from build123d import *

# Parameters (mm, degrees)
BOSS_EXTRUDE1_DEPTH     = 80
CUT_EXTRUDE1_DEPTH      = 206.243757518
CUT_EXTRUDE1_DEPTH_BACK = 206.243757518
SKETCH2_R               = 4
SKETCH5_W               = 15
SKETCH5_H               = 15
BOSS_EXTRUDE2_DEPTH     = 90
CUT_EXTRUDE2_DEPTH      = 230
CUT_EXTRUDE2_DEPTH_BACK = 10
SKETCH6_R               = 4
CUT_EXTRUDE3_DEPTH      = 80
CUT_EXTRUDE3_DEPTH_BACK = 90
SKETCH8_W               = 15
SKETCH8_H               = 23
BOSS_EXTRUDE3_DEPTH     = 15
FILLET1_R               = 10
FILLET2_R               = 10
CUT_EXTRUDE5_DEPTH      = 245
CUT_EXTRUDE5_DEPTH_BACK = 278.173231031
SKETCH9_R               = 2
SKETCH11_W              = 3.463440771
SKETCH11_H              = 73
SKETCH11_W_2            = 3
SKETCH11_H_2            = 54.709634628
BOSS_EXTRUDE4_DEPTH     = 10


with BuildPart() as part:
    # Sketch1 → Boss-Extrude1 (new body)
    with BuildSketch(Plane(origin=(0, 0, 0), x_dir=(1, 0, 0), z_dir=(0, 1, 0))):
        Polygon((-115, 150), (115, 150), (115, -150), (75, -107.115172571), (75, 147), (-75, 147), (-77, 147), (-77, 142.176566344), (-112, 142.176566344), (-112, -92.757359313), (-75, -92.757359313), (-75, -107.115172571), (-115, -150), (-115, -147), (-115, -92.757359313), (-115, 147), align=None)
        Polygon((112, 147), (112, -112), (112, -143.851442339), (77, -106.327218338), (77, 147), align=None, mode=Mode.SUBTRACT)
        Polygon((-112, -112), (-112, -143.851442339), (-77, -106.327218338), (-77, -99.920571676), (-112, -99.920571676), align=None, mode=Mode.SUBTRACT)
    extrude(amount=BOSS_EXTRUDE1_DEPTH)

    # Sketch2 → Cut-Extrude1 (cut, two sides: drawn at the far end of the back side and taken through both)
    with BuildSketch(Plane(origin=(0, 0, 0), x_dir=(0, 0, -1), z_dir=(1, 0, 0)).offset(-CUT_EXTRUDE1_DEPTH_BACK)):
        with Locations((90, 28)):
            Circle(SKETCH2_R)
        with Locations((-30, 28)):
            Circle(SKETCH2_R)
    extrude(amount=CUT_EXTRUDE1_DEPTH + CUT_EXTRUDE1_DEPTH_BACK, mode=Mode.SUBTRACT)

    # Sketch5 → Boss-Extrude2 (add)
    with BuildSketch(Plane(origin=(0, 0, 0), x_dir=(1, 0, 0), z_dir=(0, 1, 0))):
        Polygon((-115, -127), (-100, -127), (-100, -135), (-115, -150), (-115, -140.427238406), align=None)
        Polygon((115, -150), (100, -135), (100, -127), (115, -127), (115, -140.427238406), align=None)
        with Locations((107.5, 142.5)):
            Rectangle(SKETCH5_W, SKETCH5_H)
        with Locations((-107.5, 142.5)):
            Rectangle(SKETCH5_W, SKETCH5_H)
    extrude(amount=BOSS_EXTRUDE2_DEPTH)

    # Sketch6 → Cut-Extrude2 (cut, two sides: drawn at the far end of the back side and taken through both)
    with BuildSketch(Plane(origin=(-112, 0, 0), x_dir=(0, 0, -1), z_dir=(1, 0, 0)).offset(-CUT_EXTRUDE2_DEPTH_BACK)):
        with Locations((76, 17)):
            Circle(SKETCH6_R)
        with Locations((104, 17)):
            Circle(SKETCH6_R)
        with Locations((104, 57)):
            Circle(SKETCH6_R)
        with Locations((76, 57)):
            Circle(SKETCH6_R)
        with Locations((-16, 57)):
            Circle(SKETCH6_R)
        with Locations((-44, 57)):
            Circle(SKETCH6_R)
        with Locations((-44, 17)):
            Circle(SKETCH6_R)
        with Locations((-16, 17)):
            Circle(SKETCH6_R)
    extrude(amount=CUT_EXTRUDE2_DEPTH + CUT_EXTRUDE2_DEPTH_BACK, mode=Mode.SUBTRACT)

    # Sketch7 → Cut-Extrude3 (cut, two sides: drawn at the far end of the back side and taken through both)
    with BuildSketch(Plane(origin=(0, 0, 0), x_dir=(0, 0, -1), z_dir=(1, 0, 0)).offset(-CUT_EXTRUDE3_DEPTH_BACK)):
        Polygon((-127, 80), (-127, 49.75530595), (136.100135801, 49.75530595), (135, 80), align=None)
    extrude(amount=CUT_EXTRUDE3_DEPTH + CUT_EXTRUDE3_DEPTH_BACK, mode=Mode.SUBTRACT)

    # Sketch8 → Boss-Extrude3 (add)
    with BuildSketch(Plane(origin=(0, 90, 0), x_dir=(1, 0, 0), z_dir=(0, 1, 0))):
        with Locations((107.5, -138.5)):
            Rectangle(SKETCH8_W, SKETCH8_H)
        with Locations((-107.5, -138.5)):
            Rectangle(SKETCH8_W, SKETCH8_H)
    extrude(amount=-BOSS_EXTRUDE3_DEPTH)

    # Fillet1
    fillet1_edges = [part.edges().sort_by_distance(p)[0] for p in [
        (107.5, 75, 142.5),
    ]]
    fillet(fillet1_edges, radius=FILLET1_R)

    # Fillet2
    fillet2_edges = [part.edges().sort_by_distance(p)[0] for p in [
        (-107.5, 75, 142.5),
    ]]
    fillet(fillet2_edges, radius=FILLET2_R)

    # Sketch9 → Cut-Extrude5 (cut, two sides: drawn at the far end of the back side and taken through both)
    with BuildSketch(Plane.ZY.offset(-100).offset(-CUT_EXTRUDE5_DEPTH_BACK)):
        with Locations(Location((138.5, 77.5, 0), (0, 0, 180))):
            Circle(SKETCH9_R)
    extrude(amount=CUT_EXTRUDE5_DEPTH + CUT_EXTRUDE5_DEPTH_BACK, mode=Mode.SUBTRACT)

    # Sketch11 → Boss-Extrude4 (add, through all)
    with BuildSketch(Plane(origin=(0, 80, 0), x_dir=(1, 0, 0), z_dir=(0, 1, 0))):
        with Locations((-113.268279615, 28.5)):
            Rectangle(SKETCH11_W, SKETCH11_H)
        with Locations((113.5, 28.5)):
            Rectangle(SKETCH11_W_2, SKETCH11_H)
        with Locations((-113.5, -82.354817314)):
            Rectangle(SKETCH11_W_2, SKETCH11_H_2)
        with Locations((113.5, -82.354817314)):
            Rectangle(SKETCH11_W_2, SKETCH11_H_2)
    extrude(amount=BOSS_EXTRUDE4_DEPTH)


solid = part.part
Geometry: final body of the model. Coordinates: model frame, mm. A direction names the side the tool comes from. Coordinates: 2 decimals unless noted, no trailing zeros. Order: outer loops, then holes, each group sorted by start corner. A loop starts at its lowest first (then second) coordinate and runs counter-clockwise, first axis right, second up.
(1) Section query C-C (x = -33.5). Return the cut outline in (y, z).
(2) Material intervals for probe 1 along X at (y, z) = (10, 68); probe 2 along Y at (x, z) = (-114.35, -76); probe 3 along Z at (x, y) = (106.5, 77.5), sorted ascending.
(3) First-contact query: pin 1 (8 mm diameter, centred on x = -96.5, z = 130, fed in from +Y); pin 2 (4 mm diameter, centred on x = 77.5, z = -70, fed in from +Y); pin 3 (17.5 mm diameter, centred on x = -92.5, y = 51, fed in from +Z); pin 4 (2 mm diameter, centred on x = 23, y = 60, fed in from +Z). Flat tips, straight axial feed; report the tip coordinate or a pass-through.
(4) Section query B-B (z = -76). State how many separate pieces and enclosed holes the cut face has, plus the area to 3 significant figures.
(5) Draft query along Y for faces 1 (the face through (113.479, 53.095, 44.867)), 2 (the face through (115, 44, -2)), 3 (the face through (107, 90, 138)). Return one class per face: pulls with the +Y half, pulls with the -Y half, needs draft (parallel to the pull), parting line crosses it, or undercut.
(6) Section query A-A (z = -30.5). Return the cut outline in (x, y), plus the area to 3 significant figures.
(7) Access query for faces 4 (the face through (90, 80, 122)), 5 (the face through (-101, 80, 96)), 6 (the face through (-77, 25, 103)). Directions: +Z, -Z, +X, -X, +Y, -Y. A direction counts if a zero-diameter tool reaches every point of the face in a straight line with its end or side. Return the directions, or none.
Solution:
1. outline: (0, -150) - (80, -150) - (80, -147) - (0, -147) - close
2. probe 1: x = -115 to -112, 75 to 77, 112 to 115
2. probe 2: y = 0 to 13, 21 to 53, 61 to 80
2. probe 3: z = -150 to -135, 127 to 136.5, 140.5 to 150
3. pin 1: stops at y = 90
3. pin 2: stops at y = 49.76
3. pin 3: stops at z = 136.25
3. pin 4: stops at z = -147
4. separate pieces: 8
4. enclosed holes: 0
4. area: 468 mm2
5. face 1: undercut
5. face 2: needs draft
5. face 3: pulls with the +Y half
6. outline: (-115, 0) - (-112, 0) - (-112, 80) - (-111.54, 80) - (-111.54, 90) - (-115, 90) - close; (75, 0) - (77, 0) - (77, 49.76) - (75, 49.76) - close; (112, 0) - (115, 0) - (115, 90) - (112, 90) - close
6. area: 644 mm2
7. face 4: +Z, -Z, +Y
7. face 5: +Y
7. face 6: +Y, -Y
